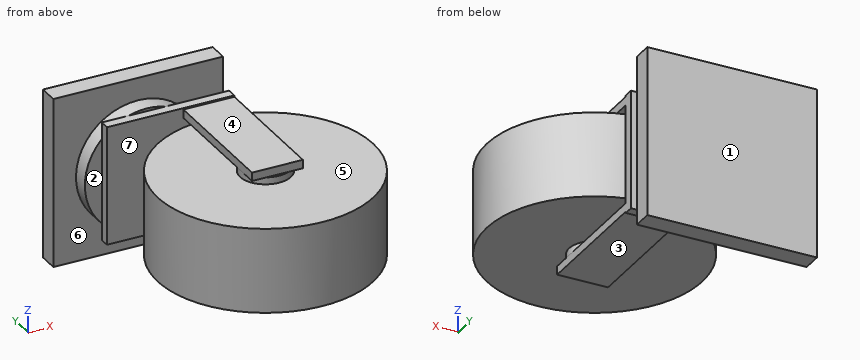
```python
from build123d import *

# Parameters (mm, degrees)
P01_SPACER4MM_START  = 89
SK_P01_SPACER4MM_W   = 60
SK_P01_SPACER4MM_H   = 60
P01_SPACER4MM_DEPTH  = 4
P02_TOPPLATE_START   = 86
SK_P02_TOPPLATE_W    = 60
SK_P02_TOPPLATE_H    = 60
P02_TOPPLATE_DEPTH   = 3
P03_SWIVELRACE_START = 80
SK_P03_SWIVELRACE_R  = 22
P03_SWIVELRACE_DEPTH = 6
P04_FORKYOKE_START   = 76.5
SK_P04_FORKYOKE_W    = 45
SK_P04_FORKYOKE_H    = 42
P04_FORKYOKE_DEPTH   = 3.5
P05_FORKLEG_START    = 30
SK_P05_FORKLEG_W     = 18
SK_P05_FORKLEG_H     = 3
P05_FORKLEG_DEPTH    = 48
P06_FORKLEG_START    = 30
SK_P06_FORKLEG_W     = 18
SK_P06_FORKLEG_H     = 3
P06_FORKLEG_DEPTH    = 48
P07_WHEEL3IN_START   = -15
SK_P07_WHEEL3IN_R    = 38.1
P07_WHEEL3IN_DEPTH   = 30
P08_AXLE_START       = -17.5
SK_P08_AXLE_R        = 9
P08_AXLE_DEPTH       = 35


with BuildPart() as part:
    # SK_P01_Spacer4mm → P01_Spacer4mm (new body)
    with BuildSketch(Plane(origin=(0, 0, 0), x_dir=(1, 0, 0), z_dir=(0, 1, 0)).offset(P01_SPACER4MM_START)):
        with Locations((-14.05, 0)):
            Rectangle(SK_P01_SPACER4MM_W, SK_P01_SPACER4MM_H)
    extrude(amount=P01_SPACER4MM_DEPTH)

    # SK_P02_Topplate → P02_Topplate (add)
    with BuildSketch(Plane(origin=(0, 0, 0), x_dir=(1, 0, 0), z_dir=(0, 1, 0)).offset(P02_TOPPLATE_START)):
        with Locations((-14.05, 0)):
            Rectangle(SK_P02_TOPPLATE_W, SK_P02_TOPPLATE_H)
    extrude(amount=P02_TOPPLATE_DEPTH)

    # SK_P03_Swivelrace → P03_Swivelrace (add)
    with BuildSketch(Plane(origin=(0, 0, 0), x_dir=(1, 0, 0), z_dir=(0, 1, 0)).offset(P03_SWIVELRACE_START)):
        with Locations(Location((-14.05, 0, 0), (0, 0, 270))):
            Circle(SK_P03_SWIVELRACE_R)
    extrude(amount=P03_SWIVELRACE_DEPTH)

    # SK_P04_Forkyoke → P04_Forkyoke (add)
    with BuildSketch(Plane(origin=(0, 0, 0), x_dir=(1, 0, 0), z_dir=(0, 1, 0)).offset(P04_FORKYOKE_START)):
        with Locations((-7.55, 0)):
            Rectangle(SK_P04_FORKYOKE_W, SK_P04_FORKYOKE_H)
    extrude(amount=P04_FORKYOKE_DEPTH)

    # SK_P05_Forkleg → P05_Forkleg (add)
    with BuildSketch(Plane(origin=(0, 0, 0), x_dir=(1, 0, 0), z_dir=(0, 1, 0)).offset(P05_FORKLEG_START)):
        with Locations((5.95, 19)):
            Rectangle(SK_P05_FORKLEG_W, SK_P05_FORKLEG_H)
    extrude(amount=P05_FORKLEG_DEPTH)

    # SK_P06_Forkleg → P06_Forkleg (add)
    with BuildSketch(Plane(origin=(0, 0, 0), x_dir=(1, 0, 0), z_dir=(0, 1, 0)).offset(P06_FORKLEG_START)):
        with Locations((5.95, -19)):
            Rectangle(SK_P06_FORKLEG_W, SK_P06_FORKLEG_H)
    extrude(amount=P06_FORKLEG_DEPTH)



with BuildPart() as body_2:
    # SK_P07_Wheel3in → P07_Wheel3in (new body)
    with BuildSketch(Plane.XY.offset(P07_WHEEL3IN_START)):
        with Locations((5.95, 38.1)):
            Circle(SK_P07_WHEEL3IN_R)
    extrude(amount=P07_WHEEL3IN_DEPTH)


with BuildPart() as part_1:
    add(part.part)

    add(body_2.part)  # P08_Axle merges body 2
    # SK_P08_Axle → P08_Axle (add)
    with BuildSketch(Plane.XY.offset(P08_AXLE_START)):
        with Locations((5.95, 38.1)):
            Circle(SK_P08_AXLE_R)
    extrude(amount=P08_AXLE_DEPTH)


solid = part_1.part
```
Model file for the job. Use its own axes, mm. Face numbers are marked on the shaded views. A direction names the side the tool comes from. Coordinates: 2 decimals unless noted, no trailing zeros. Order: outer loops, then holes, each group sorted by start corner. A loop starts at its lowest first (then second) coordinate and runs counter-clockwise, first axis right, second up. Notation, with made-up numbers: (-19.5, -28.75) -> (37.5, -28.75) arc R12 ccw to (37.5, -12.75) -> close; hole circle Ø3 at (-14, 4). An arc over 180 degrees is marked (long way). Return JSON: item names as keys, results as strings.
Item 1: Slice it at D-D (x = -14.05). Write the cut outline in (y, z), then the cut area to 3 significant figures.
Model answer:
{"outline": "(5.67, -15) -> (70.53, -15) -> (70.53, 15) -> (5.67, 15) -> close; (76.5, -21) -> (80, -21) -> (80, -22) -> (86, -22) -> (86, -30) -> (93, -30) -> (93, 30) -> (86, 30) -> (86, 22) -> (80, 22) -> (80, 21) -> (76.5, 21) -> close", "area": "2,780 mm²"}
Item 2: 3-axis set-ups, long thin cutter, end or side, ignore diameter. For the marked faces 1, 2 and 3: which of +Z, -Z, +X, -X, +Y, -Y reach the whole face in a straight line?
Model answer:
{"face 1": "+Z, -Z, +X, -X, +Y", "face 2": "+Z, -Z, -X", "face 3": "-Z, +X, -X, -Y"}
Item 3: Slice it at A-A (z = 0). Write the cut outline in (x, y).
Model answer:
{"outline": "(-44.05, 86) -> (-36.05, 86) -> (-36.05, 80) -> (-30.05, 80) -> (-30.05, 76.5) -> (14.95, 76.5) -> (14.95, 80) -> (7.95, 80) -> (7.95, 86) -> (15.95, 86) -> (15.95, 93) -> (-44.05, 93) -> close; circle Ø76.2 at (5.95, 38.1)"}
Item 4: Wall check: line 1 along Z through (x, y) = (0.5, 57.5); line 2 along X through (y, z) = (39.5, -14.5); line 3 along Y through (x, z) = (0, 16). Give the ranges that are in metal, low to high. Write a range as from..to.
Model answer:
{"line 1": "z = -20.5..-17.5, -15..15, 17.5..20.5", "line 2": "x = -32.12..44.02", "line 3": "y = 31.35..44.85, 76.5..93"}
Item 5: Pin check, flat tips, straight feed: P1, Ø4, axis at x = -20.5, y = 59, coming from the -Z side; P2, Ø8, axis at x = 0.5, z = -15.5, coming from the -Y side; P3, Ø1.5, axis at x = 13.5, y = 34, coming from the -Z side. Stop position of each tip, or through.
Model answer:
{"P1": "stops at z = -15", "P2": "stops at y = 0.03", "P3": "stops at z = -20.5"}
Item 6: Mould opens along Z. For the marked faces 4, 5, 6 and 7 say: pulls with the +Z half, pulls with the -Z half, needs draft (parallel to the pull), parting line crosses it, or undercut.
Model answer:
{"face 4": "pulls with the +Z half", "face 5": "undercut", "face 6": "needs draft", "face 7": "undercut"}
Item 7: Slice it at C-C (y = 54). Write the cut outline in (x, z), then the cut area to 3 significant figures.
Model answer:
{"outline": "(-28.67, -15) -> (40.57, -15) -> (40.57, 15) -> (-28.67, 15) -> close; (-3.05, -20.5) -> (14.95, -20.5) -> (14.95, -17.5) -> (-3.05, -17.5) -> close; (-3.05, 17.5) -> (14.95, 17.5) -> (14.95, 20.5) -> (-3.05, 20.5) -> close", "area": "2,190 mm²"}
